from build123d import *

# Parameters (mm, degrees)
SKETCH_1_R          = 6.25
EXTRUDE_1_DEPTH     = 10
SKETCH_2_R          = 3.5
CUT_EXTRUDE_2_DEPTH = 53.440442409
SKETCH_3_R          = 3.5
CUT_EXTRUDE_3_DEPTH = 53.440442409


with BuildPart() as part:
    # 草圖1 → 填料-伸長1 (new body)
    with BuildSketch(Plane.XY):
        Polygon((30, 0), (45, 0), (45, -8), (-15, -8), (-15, 0), (0, 0), (0, 25), (30, 25), align=None)
        with Locations((15, 12)):
            Circle(SKETCH_1_R, mode=Mode.SUBTRACT)
    extrude(amount=EXTRUDE_1_DEPTH)

    # 草圖2 → 除料-伸長2 (cut, through all)
    with BuildSketch(Plane(origin=(0, 0, 0), x_dir=(1, 0, 0), z_dir=(0, 1, 0))):
        with Locations(Location((37.5, -5, 0), (0, 0, 270))):
            Circle(SKETCH_2_R)
    extrude(amount=-CUT_EXTRUDE_2_DEPTH, mode=Mode.SUBTRACT)

    # 草圖3 → 除料-伸長3 (cut, through all)
    with BuildSketch(Plane(origin=(0, 0, 0), x_dir=(1, 0, 0), z_dir=(0, 1, 0))):
        with Locations(Location((-7.5, -5, 0), (0, 0, 270))):
            Circle(SKETCH_3_R)
    extrude(amount=-CUT_EXTRUDE_3_DEPTH, mode=Mode.SUBTRACT)


solid = part.part
Could you check a few things on this model? Use its own coordinates, in mm. A direction names the side the tool comes from. Coordinates: 2 decimals unless noted, no trailing zeros. Loops run counter-clockwise (first coordinate to the right, second up) from the corner with the lowest first, then second, coordinate; pieces in that order, holes last. Notation, with made-up numbers: (-23, -12) -> (-4, -12) arc R30 ccw to (-4, 20) -> close; hole circle Ø2 at (24.5, 86.25). An arc over 180 degrees is marked (long way). Answer in a Markdown table with one row per item.
(1) Imagine slicing it at C-C (y = 12). List the corners of the cut face in (x, z) for me, plus the area to 3 significant figures.
Results found:
| item | result |
|---|---|
| outline | (0, 0) -> (8.75, 0) -> (8.75, 10) -> (0, 10) -> close; (21.25, 0) -> (30, 0) -> (30, 10) -> (21.25, 10) -> close |
| area | 175 mm^2 |
(2) Imagine slicing it at A-A (z = 5). List the corners of the cut face in (x, y) for me, plus the area to 3 significant figures.
Results found:
| item | result |
|---|---|
| outline | (-15, -8) -> (-11, -8) -> (-11, 0) -> (-15, 0) -> close; (-4, -8) -> (34, -8) -> (34, 0) -> (30, 0) -> (30, 25) -> (0, 25) -> (0, 0) -> (-4, 0) -> close; (41, -8) -> (45, -8) -> (45, 0) -> (41, 0) -> close; hole circle Ø12.5 at (15, 12) |
| area | 995 mm^2 |
(3) Imagine slicing it at B-B (x = -7.5). List the corners of the cut face in (y, z) for me.
Results found:
| item | result |
|---|---|
| outline | (-8, 0) -> (0, 0) -> (0, 1.5) -> (-8, 1.5) -> close; (-8, 8.5) -> (0, 8.5) -> (0, 10) -> (-8, 10) -> close |
(4) If I drill on probe 1 along X at (y, z) = (-4.25, 5); probe 2 along Y at (x, z) = (15, 8.25); probe 3 along Y at (x, z) = (34.5, 7.25), over which ranges is the centre line in solid material (lowest first)?
Results found:
| item | result |
|---|---|
| probe 1 | x = -15 to -11, -4 to 34, 41 to 45 |
| probe 2 | y = -8 to 5.75, 18.25 to 25 |
| probe 3 | y = -8 to 0 |
(5) For faces 4 (the face through (35.7, 0, 1.6)), 5 (the face through (0, 12, 5)), 6 (the face through (-15, -4, 5)), which set-ups out of +Z, -Z, +X, -X, +Y, -Y let a thin tool reach every point of the face, with its end or its side?
Results found:
| item | result |
|---|---|
| face 4 | +Z, -Z, +X, +Y |
| face 5 | +Z, -Z, -X, +Y |
| face 6 | +Z, -Z, -X, +Y, -Y |
(6) Thinking about a two-plate mould opening in X: for faces 1 (the face through (15, 25, 5)), 2 (the face through (41, -4, 5)), 3 (the face through (30, 13, 5)), which applies, released by +X, released by -X, zero draft, split by the parting line, or undercut?
Results found:
| item | result |
|---|---|
| face 1 | zero draft |
| face 2 | undercut |
| face 3 | released by +X |
(7) Will these pins go through, and if not, where does the flat tip stop? pin 1 Ø1.5 at (x, z) = (38, 4) entering from +Y; pin 2 Ø3 at (y, z) = (15.5, 4) entering from -X; pin 3 Ø3 at (y, z) = (16.5, 6) entering from +X.
Results found:
| item | result |
|---|---|
| pin 1 | passes through |
| pin 2 | stops at x = 0 |
| pin 3 | stops at x = 30 |
(8) Imagine slicing it at D-D (y = -3). List the corners of the cut face in (x, z) for me.
Results found:
| item | result |
|---|---|
| outline | (-15, 0) -> (45, 0) -> (45, 10) -> (-15, 10) -> close; hole circle Ø7 at (-7.5, 5); hole circle Ø7 at (37.5, 5) |
